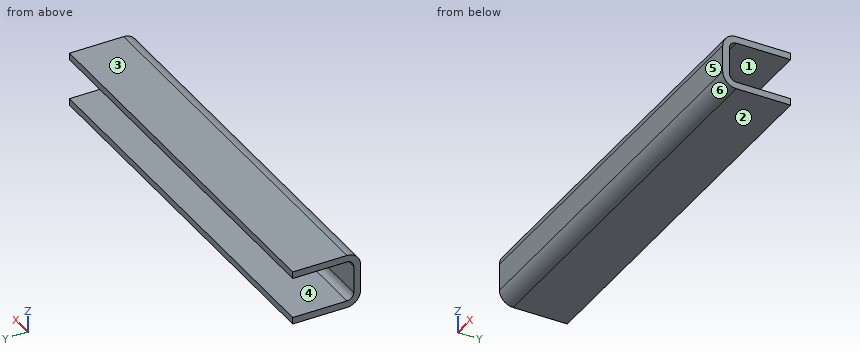
```python
from build123d import *

# Parameters (mm, degrees)
TUBO_RECTANGULAR_3_X_2_X_0_25_1_DEPTH = 375
CROQUIS3_W                            = 375
CROQUIS3_H                            = 12.7
CORTAR_EXTRUIR1_DEPTH                 = 78


with BuildPart() as part:
    # Sketch1 → Tubo rectangular 3 X 2 X 0.25(1) (new body)
    with BuildSketch(Plane(origin=(0, 0, 0), x_dir=(0, 0, -1), z_dir=(1, 0, 0))):
        with BuildLine():
            Line((-12.699978, -38.1), (12.699978, -38.1))
            ThreePointArc((12.699978, -38.1), (21.680234121, -34.380256121), (25.399978, -25.4))
            Line((25.399978, -25.4), (25.399978, 25.4))
            ThreePointArc((25.399978, 25.4), (21.680234121, 34.380256121), (12.699978, 38.1))
            Line((12.699978, 38.1), (-12.699978, 38.1))
            ThreePointArc((-12.699978, 38.1), (-21.680234121, 34.380256121), (-25.399978, 25.4))
            Line((-25.399978, 25.4), (-25.399978, -25.4))
            ThreePointArc((-25.399978, -25.4), (-21.680234121, -34.380256121), (-12.699978, -38.1))
        make_face()
        with BuildLine():
            Line((-12.699978, -31.75), (12.699978, -31.75))
            ThreePointArc((12.699978, -31.75), (17.190106061, -29.890128061), (19.049978, -25.4))
            Line((19.049978, -25.4), (19.049978, 25.4))
            ThreePointArc((19.049978, 25.4), (17.190106061, 29.890128061), (12.699978, 31.75))
            Line((12.699978, 31.75), (-12.699978, 31.75))
            ThreePointArc((-12.699978, 31.75), (-17.190106061, 29.890128061), (-19.049978, 25.4))
            Line((-19.049978, 25.4), (-19.049978, -25.4))
            ThreePointArc((-19.049978, -25.4), (-17.190106061, -29.890128061), (-12.699978, -31.75))
        make_face(mode=Mode.SUBTRACT)
    extrude(amount=TUBO_RECTANGULAR_3_X_2_X_0_25_1_DEPTH)

    # Croquis3 → Cortar-Extruir1 (cut)
    with BuildSketch(Plane(origin=(0, 0, -25.399978), x_dir=(-1, 0, 0), z_dir=(0, 0, -1))):
        with Locations((-187.5, 31.75)):
            Rectangle(CROQUIS3_W, CROQUIS3_H)
    extrude(amount=-CORTAR_EXTRUIR1_DEPTH, mode=Mode.SUBTRACT)


solid = part.part
```
Verification items for the finished model (mm, model axes). Face numbers are marked on the shaded views. A direction names the side the tool comes from. Coordinates: 2 decimals unless noted, no trailing zeros. Loops run counter-clockwise (first coordinate to the right, second up) from the corner with the lowest first, then second, coordinate; pieces in that order, holes last. Notation, with made-up numbers: (23.5, 19.25) - (59.5, 19.25) arc R21 ccw to (59.5, 28.25) - close; hole circle Ø4 at (46, 41.25). An arc over 180 degrees is marked (long way). Answer as a JSON object with one key per item and string values.
(1) Go/stop test with flat-tipped pins: pin 1 Ø10 at (x, z) = (98.5, -9.5) entering from +Y; pin 2 Ø5 at (y, z) = (6.5, -16.5) entering from -X; pin 3 Ø5 at (x, z) = (213.5, 19.5) entering from -Y; pin 4 Ø5 at (y, z) = (-1, -19.5) entering from -X. Record where each tip stops, or that it passes through.
Response:
{"pin 1": "stops at y = -31.49", "pin 2": "passes through", "pin 3": "stops at y = -37.35", "pin 4": "stops at x = 0"}
(2) Mould release check, pull along Z, two halves, no side actions. Record for the marked faces 3, 4, 5 and 6: pulls with the +Z half, pulls with the -Z half, needs draft (parallel to the pull), parting line crosses it, or undercut.
Response:
{"face 3": "pulls with the +Z half", "face 4": "undercut", "face 5": "needs draft", "face 6": "pulls with the -Z half"}
(3) Cross-section at B-B, the plane x = 254.5. Record the boundary of the cut face in (y, z).
Response:
{"outline": "(-38.1, -12.7) arc R12.7 ccw to (-25.4, -25.4) - (25.4, -25.4) - (25.4, -19.05) - (-25.4, -19.05) arc R6.35 cw to (-31.75, -12.7) - (-31.75, 12.7) arc R6.35 cw to (-25.4, 19.05) - (25.4, 19.05) - (25.4, 25.4) - (-25.4, 25.4) arc R12.7 ccw to (-38.1, 12.7) - close"}
(4) Access from +Z, -Z, +X, -X, +Y, -Y to the whole of each face (thin tool, end or side, straight path). Record for the marked faces 1 and 2.
Response:
{"face 1": "+X, -X, +Y", "face 2": "-Z, +X, -X, +Y, -Y"}
(5) Cross-section at A-A, the plane y = -1. Record the boundary of the cut face in (x, z), then the cut area to 3 significant figures.
Response:
{"outline": "(0, -25.4) - (375, -25.4) - (375, -19.05) - (0, -19.05) - close; (0, 19.05) - (375, 19.05) - (375, 25.4) - (0, 25.4) - close", "area": "4,760 mm²"}
(6) Scan lines: line 1 along Z through (x, y) = (282.5, 4); line 2 along Y through (x, z) = (309, -12); line 3 along Z through (x, y) = (273, -30.5). Record each from-to range of solid material in increasing order.
Response:
{"line 1": "z = -25.4 to -19.05, 19.05 to 25.4", "line 2": "y = -38.1 to -31.75", "line 3": "z = -24.33 to -16.48, 16.48 to 24.33"}
(7) Cross-section at C-C, the plane z = 0.5. Record the boundary of the cut face in (x, y), then the cut area to 3 significant figures.
Response:
{"outline": "(0, -38.1) - (375, -38.1) - (375, -31.75) - (0, -31.75) - close", "area": "2,380 mm²"}
